```python
from build123d import *

# Parameters (mm, degrees)
SKETCH1_R                 = 6.35
BOSS_EXTRUDE1_DEPTH       = 12.7
F_1_4_20_TAPPED_HOLE1_D   = 5.1054
F_6_32_TAPPED_HOLE1_D     = 2.7051
F_6_32_TAPPED_HOLE1_DEPTH = 9.398
F_6_32_TAPPED_HOLE1_TIP   = 0.81269403


with BuildPart() as part:
    # Sketch1 → Boss-Extrude1 (new body)
    with BuildSketch(Plane.XY):
        with BuildLine():
            Line((38.1, 12.7), (38.1, 25.4))
            ThreePointArc((38.1, 25.4), (30.260079591, 37.133270063), (16.419743879, 34.380256121))
            Line((16.419743879, 34.380256121), (-3.772614691, 14.187897552))
            ThreePointArc((-3.772614691, 14.187897552), (-5.420685303, 13.086691975), (-7.364717139, 12.7))
            Line((-7.364717139, 12.7), (-20.32, 12.7))
            Line((-20.32, 12.7), (-20.32, 11.43))
            ThreePointArc((-20.32, 11.43), (-20.691974388, 10.531974388), (-21.59, 10.16))
            Line((-21.59, 10.16), (-29.21, 10.16))
            ThreePointArc((-29.21, 10.16), (-30.108025612, 10.531974388), (-30.48, 11.43))
            Line((-30.48, 11.43), (-30.48, 12.7))
            Line((-30.48, 12.7), (-38.1, 12.7))
            Line((-38.1, 12.7), (-38.1, -12.7))
            Line((-38.1, -12.7), (38.1, -12.7))
            Line((38.1, -12.7), (38.1, 12.7))
        make_face()
        with Locations((25.4, 25.4)):
            Circle(SKETCH1_R, mode=Mode.SUBTRACT)
    extrude(amount=BOSS_EXTRUDE1_DEPTH)

    # 1/4-20 Tapped Hole1 (through all)
    with Locations(Plane.XY.offset(12.7)):
        with Locations((-15.24, -2.54), (5.08, -2.54), (25.4, -2.54)):
            Hole(F_1_4_20_TAPPED_HOLE1_D / 2)

    # #6-32 Tapped Hole1
    with Locations(Plane(origin=(0, 10.16, 0), x_dir=(1, 0, 0), z_dir=(0, 1, 0))):
        with Locations((-25.4, -6.35)):
            Hole(F_6_32_TAPPED_HOLE1_D / 2, depth=F_6_32_TAPPED_HOLE1_DEPTH)
            with Locations((0, 0, -(F_6_32_TAPPED_HOLE1_DEPTH + F_6_32_TAPPED_HOLE1_TIP / 2))):  # 118° drill point
                Cone(0, F_6_32_TAPPED_HOLE1_D / 2, F_6_32_TAPPED_HOLE1_TIP, mode=Mode.SUBTRACT)


solid = part.part
```
Can you work these out from the model? Positions are in its coordinate system, mm. A direction names the side the tool comes from. Coordinates: 2 decimals unless noted, no trailing zeros. Loops run counter-clockwise (first coordinate to the right, second up) from the corner with the lowest first, then second, coordinate; pieces in that order, holes last. Notation, with made-up numbers: (-17.75, 31.25) -> (14.25, 31.25) arc R25 ccw to (14.25, 52.25) -> close; hole circle Ø6 at (-16, -9). An arc over 180 degrees is marked (long way). Answer as a JSON object with one key per item and string values.
1) Imagine slicing it at C-C (y = -3.5). Please give me the cut outline in (x, z).
Results:
{"outline": "(-38.1, 0) -> (-17.61, 0) -> (-17.61, 12.7) -> (-38.1, 12.7) -> close; (-12.87, 0) -> (2.71, 0) -> (2.71, 12.7) -> (-12.87, 12.7) -> close; (7.45, 0) -> (23.03, 0) -> (23.03, 12.7) -> (7.45, 12.7) -> close; (27.77, 0) -> (38.1, 0) -> (38.1, 12.7) -> (27.77, 12.7) -> close"}
2) For faces 4 (the face through (-24.05, 5.4, 6.29)), 5 (the face through (8, 7, 0)), 6 (the face through (20.36, 21.54, 6.26)), 7 (the face through (-34, 12.7, 6)), 8 (the face through (-25.3, 10.16, 4.8)), which set-ups out of +Z, -Z, +X, -X, +Y, -Y let a thin tool reach every point of the face, with its end or its side?
Results:
{"face 4": "+Y", "face 5": "-Z, +X, -X, +Y, -Y", "face 6": "+Z, -Z", "face 7": "+Z, -Z, -X, +Y", "face 8": "+Z, -Z, +Y"}
3) Imagine slicing it at D-D (x = 5.08). Please give me the cut outline in (y, z), then the cut area to 3 significant figures.
Results:
{"outline": "(-12.7, 0) -> (-5.09, 0) -> (-5.09, 12.7) -> (-12.7, 12.7) -> close; (0.01, 0) -> (23.04, 0) -> (23.04, 12.7) -> (0.01, 12.7) -> close", "area": "389 mm^2"}
4) If I drill on line 1 (Y direction, x = 25.4, z = 6.5); line 2 (Y direction, x = -15.24, z = 8); line 3 (Y direction, x = 23.5, z = 9.5), over which ranges is the centre line in solid material (lowest first)?
Results:
{"line 1": "y = -12.7 to -5.09, 0.01 to 19.05, 31.75 to 38.1", "line 2": "y = -12.7 to -5.09, 0.01 to 12.7", "line 3": "y = -12.7 to -4.24, -0.84 to 19.34, 31.46 to 37.96"}
5) For P1, Ø6, axis at y = 26, z = 3.5, coming from the +X side; P2, Ø4, axis at x = -24, z = 8, coming from the +Y side; P3, Ø2.5, axis at x = -36, z = 9.5, coming from the +Y side, each with a flat end and sliding along its axis, tell me the tip position at first contact or that it passes through.
Results:
{"P1": "stops at x = 38.1", "P2": "stops at y = 10.16", "P3": "stops at y = 12.7"}
6) Thinking about a two-plate mould opening in Y: for faces 1 (the face through (2.722, -3.518, 6.261)), 2 (the face through (8, 7, 12.7)), 3 (the face through (6.465, 24.425, 6.261)), which applies, pulls with the +Y half, pulls with the -Y half, needs draft (parallel to the pull), parting line crosses it, or undercut?
Results:
{"face 1": "undercut", "face 2": "needs draft", "face 3": "pulls with the +Y half"}
7) Imagine slicing it at B-B (z = 1.5). Please give me the cut outline in (x, y), then the cut area to 3 significant figures.
Results:
{"outline": "(-38.1, -12.7) -> (38.1, -12.7) -> (38.1, 25.4) arc R12.7 ccw to (16.42, 34.38) -> (-3.77, 14.19) arc R5.08 cw to (-7.36, 12.7) -> (-20.32, 12.7) -> (-20.32, 11.43) arc R1.27 cw to (-21.59, 10.16) -> (-29.21, 10.16) arc R1.27 cw to (-30.48, 11.43) -> (-30.48, 12.7) -> (-38.1, 12.7) -> close; hole circle Ø5.11 at (-15.24, -2.54); hole circle Ø5.11 at (5.08, -2.54); hole circle Ø12.7 at (25.4, 25.4); hole circle Ø5.11 at (25.4, -2.54)", "area": "2,460 mm^2"}
8) Imagine slicing it at A-A (x = -15.24). Please give me the cut outline in (y, z).
Results:
{"outline": "(-12.7, 0) -> (-5.09, 0) -> (-5.09, 12.7) -> (-12.7, 12.7) -> close; (0.01, 0) -> (12.7, 0) -> (12.7, 12.7) -> (0.01, 12.7) -> close"}
